Verification items for the finished model (mm, model axes). Face numbers are marked on the shaded views. A direction names the side the tool comes from. Coordinates: 2 decimals unless noted, no trailing zeros. Loops run counter-clockwise (first coordinate to the right, second up) from the corner with the lowest first, then second, coordinate; pieces in that order, holes last. Notation, with made-up numbers: (-20, -10) -> (-14, -10) arc R25 ccw to (-14, 15) -> close; hole circle Ø10 at (14, 64). An arc over 180 degrees is marked (long way). Answer as a JSON object with one key per item and string values. Group by question number.
Q1. Release check for a two-part mould opening along Z. For the marked faces 3, 4 and 5 record: released by +Z, released by -Z, zero draft, split by the parting line, or undercut.
Q2. Cross-section at C-C on y = 6.25. Record the boundary of the cut face in (x, z), and give its area (3 significant figures).
Q3. Cross-section at B-B on x = 20.5. Record the boundary of the cut face in (y, z).
Q4. Scan lines: L1, parallel to X at y = 1, z = 2; L2, parallel to Z at x = 6.5, y = 1.5. Record each from-to range of solid material in increasing order.
Q5. Set-up check for the marked faces 1 and 2: record each of +Z, -Z, +X, -X, +Y, -Y from which the full face is reachable in a straight line by a thin tool's end or side.
Q6. Cross-section at A-A on z = 4. Record the boundary of the cut face in (x, y), and give its area (3 significant figures).
```python
from build123d import *

# Parameters (mm, degrees)
F0_W     = 5
F0_H     = 8
F1_DEPTH = 5
F2_W     = 38.5
F2_H     = 8
F3_DEPTH = 1
F4_W     = 38.5
F4_H     = 8
F5_DEPTH = 1


with BuildPart() as f1:
    # F0 (on Top) → F1 (new body)
    with BuildSketch(Plane.XY):
        with Locations((2.5, 4)):
            Rectangle(F0_W, F0_H)
        with Locations((12.5, 4)):
            Rectangle(F0_W, F0_H)
        with Locations((23.5, 4)):
            Rectangle(F0_W, F0_H)
        with Locations((36, 4)):
            Rectangle(F0_W, F0_H)
    extrude(amount=F1_DEPTH)

    # F2 (on Top) → F3 (join)
    with BuildSketch(Plane.XY):
        with Locations((19.25, 4)):
            Rectangle(F2_W, F2_H)
    extrude(amount=-F3_DEPTH)

    # F4 (on face) → F5 (join)
    with BuildSketch(Plane.XY.offset(5)):
        with Locations((19.25, 4)):
            Rectangle(F4_W, F4_H)
    extrude(amount=F5_DEPTH)


solid = f1.part
```
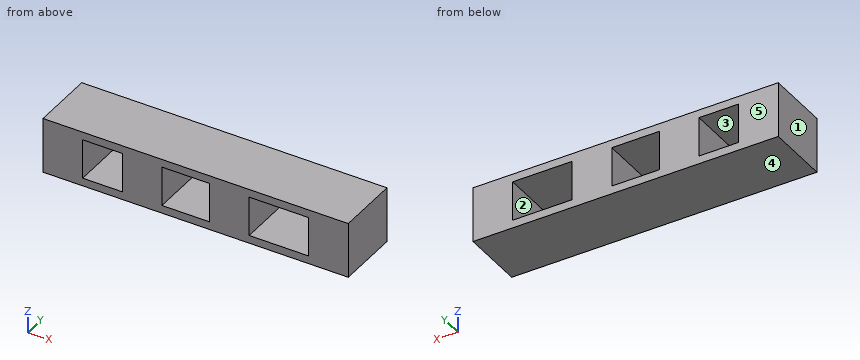
Computed values:
{
 "1": {"face 3": "undercut", "face 4": "released by -Z", "face 5": "zero draft"},
 "2": {"outline": "(0, -1) -> (38.5, -1) -> (38.5, 6) -> (0, 6) -> close; hole (5, 0) -> (10, 0) -> (10, 5) -> (5, 5) -> close; hole (15, 0) -> (21, 0) -> (21, 5) -> (15, 5) -> close; hole (26, 0) -> (33.5, 0) -> (33.5, 5) -> (26, 5) -> close", "area": "177 mm²"},
 "3": {"outline": "(0, -1) -> (8, -1) -> (8, 0) -> (0, 0) -> close; (0, 5) -> (8, 5) -> (8, 6) -> (0, 6) -> close"},
 "4": {"L1": "x = 0 to 5, 10 to 15, 21 to 26, 33.5 to 38.5", "L2": "z = -1 to 0, 5 to 6"},
 "5": {"face 1": "+Z, -Z, -X, +Y, -Y", "face 2": "+Y, -Y"},
 "6": {"outline": "(0, 0) -> (5, 0) -> (5, 8) -> (0, 8) -> close; (10, 0) -> (15, 0) -> (15, 8) -> (10, 8) -> close; (21, 0) -> (26, 0) -> (26, 8) -> (21, 8) -> close; (33.5, 0) -> (38.5, 0) -> (38.5, 8) -> (33.5, 8) -> close", "area": "160 mm²"}
}
